Can you work these out from the model? Positions are in its coordinate system, mm. A direction names the side the tool comes from. Give positions to 0.01 mm unless a question says otherwise; leave off trailing zeros. Order: outer loops, then holes, each group sorted by start corner. A loop starts at its lowest first (then second) coordinate and runs counter-clockwise, first axis right, second up. Notation, with made-up numbers: (53.5, -13.5) - (110.5, -13.5) arc R12 ccw to (110.5, -0.5) - close; hole circle Ø8 at (-13.5, 2). An arc over 180 degrees is marked (long way). Use one line per item in the form item = value. Start each with the question number.
1) Please list where these lines run through material, in increasing order: probe 1 along Y at (x, z) = (-23.5, -16); probe 2 along X at (y, z) = (8.25, -6.5); probe 3 along Z at (x, y) = (-68, 7.75) (3 decimals).
2) For pin 1 (1 mm diameter, centred on x = -73.5, y = 5, fed in from -Z); pin 2 (8 mm diameter, centred on x = -49.5, z = -24, fed in from +Y); pin 3 (2 mm diameter, centred on y = 11.5, z = -23, fed in from +X), each with a flat end and sliding along its axis, tell me the tip position at first contact or that it passes through.
3) Suppose I cut it at C-C, the plane x = -104. Write out the boundary of the cut face in (y, z) (3 decimals), and give its area (3 significant figures).
4) Suppose I cut it at B-B, the plane z = -24.5. Write out the boundary of the cut face in (x, y).
5) We'd pull the mould along Z, two halves only. Please class faces 4 (the flat face through (0, 4, -10)), 5 (the flat face through (-55, 7.7, -7.5)), 6 (the flat face through (-115, 6, -27.94)): released by +Z, released by -Z, zero draft, split by the parting line, or undercut.
6) Suppose I cut it at A-A, the plane y = 1.5. Write out the boundary of the cut face in (x, z), and give its area (3 significant figures).
7) Which directions (+Z, -Z, +X, -X, +Y, -Y) give clear straight access to the entire face, cutting with the end or side of a thin tool? Please do faces 1 (the flat face through (-114, 6, -21.59)), 2 (the flat face through (-67, 8.975, -19)), 3 (the flat face through (-54.988, 7.644, -11.466)).
8) Suppose I cut it at D-D, the plane z = -10.75. Write out the boundary of the cut face in (x, y), and give its area (3 significant figures).
```python
from build123d import *

# Parameters (mm, degrees)
BOSS_EXTRUDE1_DEPTH = 6.35
SKETCH2_W           = 5.588
SKETCH2_H           = 2.624659965
BOSS_EXTRUDE2_DEPTH = 108.458
SKETCH3_W           = 11.938
SKETCH3_H           = 6.35
BOSS_EXTRUDE3_DEPTH = 6.35
SKETCH4_R           = 1.5
CUT_EXTRUDE1_DEPTH  = 6.35
SKETCH5_W           = 24.200861289
SKETCH5_H           = 43.914531272
CUT_EXTRUDE2_DEPTH  = 6.35
BOSS_EXTRUDE8_DEPTH = 12.7
SKETCH7_R           = 1.5
CUT_EXTRUDE3_DEPTH  = 33.02
SKETCH8_W           = 11.938
SKETCH8_H           = 6.35
CUT_EXTRUDE4_DEPTH  = 33.02
CUT_EXTRUDE5_DEPTH  = 3.72534


with BuildPart() as part:
    # Sketch1 → Boss-Extrude1 (new body)
    with BuildSketch(Plane(origin=(0, 0, 0), x_dir=(1, 0, 0), z_dir=(0, 1, 0))):
        Polygon((0, 0), (0, 12.7), (11.938, 12.7), (11.938, 19.05), (-108.458, 19.05), (-108.458, 0), align=None)
    boss_extrude1 = extrude(amount=BOSS_EXTRUDE1_DEPTH)

    # Sketch2 → Boss-Extrude2 (add)
    with BuildSketch(Plane.ZY.offset(108.458)):
        with Locations((-2.794, 7.662329983)):
            Rectangle(SKETCH2_W, SKETCH2_H)
        with Locations((-16.256, 7.662329983)):
            Rectangle(SKETCH2_W, SKETCH2_H)
        Polygon((-5.588, 8.974659965), (-9.525, 6.35), (-5.588, 6.35), align=None)
        Polygon((-13.462, 6.35), (-9.525, 6.35), (-13.462, 8.974659965), align=None)
    extrude(amount=-BOSS_EXTRUDE2_DEPTH)

    # Sketch3 → Boss-Extrude3 (add)
    with BuildSketch(Plane(origin=(0, 6.35, 0), x_dir=(1, 0, 0), z_dir=(0, 1, 0))):
        with Locations((5.969, 15.875)):
            Rectangle(SKETCH3_W, SKETCH3_H)
    boss_extrude3 = extrude(amount=BOSS_EXTRUDE3_DEPTH)

    # Sketch4 → Cut-Extrude1 (cut)
    with BuildSketch(Plane(origin=(0, 0, -19.05), x_dir=(-1, 0, 0), z_dir=(0, 0, -1))):
        with Locations((-6.599652977, 4.237288993)):
            Circle(SKETCH4_R)
        with Locations((-6.263550513, 9.234799649)):
            Circle(SKETCH4_R)
    cut_extrude1 = extrude(amount=-CUT_EXTRUDE1_DEPTH, mode=Mode.SUBTRACT)

    # Mirror1: Boss-Extrude1, Boss-Extrude3, Cut-Extrude1 across plane
    add(boss_extrude1.mirror(Plane.ZY.offset(54.229)))
    add(boss_extrude3.mirror(Plane.ZY.offset(54.229)))
    add(cut_extrude1.mirror(Plane.ZY.offset(54.229)), mode=Mode.SUBTRACT)

    # Sketch5 → Cut-Extrude2 (cut)
    with BuildSketch(Plane(origin=(0, 0, -19.05), x_dir=(-1, 0, 0), z_dir=(0, 0, -1))):
        with Locations((-12.100430645, -9.257265636)):
            Rectangle(SKETCH5_W, SKETCH5_H)
    extrude(amount=-CUT_EXTRUDE2_DEPTH, mode=Mode.SUBTRACT)

    # Sketch6 → Boss-Extrude8 (add)
    with BuildSketch(Plane.XZ):
        Polygon((-108.458, -19.05), (-108.458, -21.59), (-120.396, -21.59), (-120.396, -27.94), (-108.458, -27.94), (0, -19.05), (0, -16.677943068), (-108.458, -16.677943068), align=None)
    extrude(amount=-BOSS_EXTRUDE8_DEPTH)

    # Sketch7 → Cut-Extrude3 (cut)
    with BuildSketch(Plane(origin=(0, 0, -27.94), x_dir=(-1, 0, 0), z_dir=(0, 0, -1))):
        with Locations((114.721550513, 9.234799649)):
            Circle(SKETCH7_R)
        with Locations((115.057652977, 4.237288993)):
            Circle(SKETCH7_R)
    extrude(amount=-CUT_EXTRUDE3_DEPTH, mode=Mode.SUBTRACT)

    # Sketch8 → Cut-Extrude4 (cut)
    with BuildSketch(Plane(origin=(0, 12.7, 0), x_dir=(1, 0, 0), z_dir=(0, 1, 0))):
        with Locations((-114.427, 15.875)):
            Rectangle(SKETCH8_W, SKETCH8_H)
    extrude(amount=-CUT_EXTRUDE4_DEPTH, mode=Mode.SUBTRACT)

    # Sketch9 → Cut-Extrude5 (cut)
    with BuildSketch(Plane(origin=(0, 12.7, 0), x_dir=(1, 0, 0), z_dir=(0, 1, 0))):
        Polygon((-108.458, 27.94), (-108.458, 21.59), (-108.458, 16.677943068), (0, 16.677943068), (0, 19.05), align=None)
    extrude(amount=-CUT_EXTRUDE5_DEPTH, mode=Mode.SUBTRACT)


solid = part.part
```
Result sheet:
q1.probe_1 = 0 to 8.97
q1.probe_2 = -108.46 to 0
q1.probe_3 = -24.624 to -11.625, -7.425 to 0
q2.pin_1 = -25.12
q2.pin_2 = 8.97
q2.pin_3 = -108.46
q3.outline = (0, -27.575) - (8.975, -27.575) - (8.975, -13.462) - (6.35, -9.525) - (8.975, -5.588) - (8.975, 0) - (0, 0) - close
q3.area = 237 mm²
q4.outline = (-120.4, 0) - (-66.49, 0) - (-66.49, 8.97) - (-108.46, 8.97) - (-108.46, 12.7) - (-120.4, 12.7) - close; hole circle Ø3 at (-115.06, 4.24); hole circle Ø3 at (-114.72, 9.23)
q5.face_4 = zero draft
q5.face_5 = undercut
q5.face_6 = released by -Z
q6.outline = (-120.4, -27.94) - (-108.46, -27.94) - (0, -19.05) - (0, 0) - (-108.46, 0) - (-108.46, -21.59) - (-120.4, -21.59) - close
q6.area = 2,620 mm²
q7.face_1 = +Z, -X, +Y, -Y
q7.face_2 = +Z, -Z, +X, +Y
q7.face_3 = +X, -X, +Y
q8.outline = (-108.46, 0) - (0, 0) - (0, 7.17) - (-108.46, 7.17) - close
q8.area = 777 mm²
